Part model, mm, in its own coordinate system. A direction names the side the tool comes from. Give positions to 0.01 mm unless a question says otherwise; leave off trailing zeros. Write each loop counter-clockwise with the first axis right and the second up, starting at its lowest first coordinate (ties: lowest second). Pieces come first, ordered by that corner, then holes.
```python
from build123d import *

# Parameters (mm, degrees)
EXTRUDE_THIN1_DEPTH = 756.30962295
SKETCH2_R           = 45
EXTRUDE1_DEPTH      = 3
LPATTERN1_COUNT     = 7
LPATTERN1_PITCH     = 115
LPATTERN2_COUNT     = 7
LPATTERN2_PITCH     = 115
SKETCH3_R           = 3.175
EXTRUDE2_DEPTH      = 111


with BuildPart() as part:
    # Sketch1 → Extrude-Thin1 (new body, symmetric)
    with BuildSketch(Plane.XY):
        with BuildLine():
            Line((25.4, 55), (2.54, 55))
            ThreePointArc((2.54, 55), (0.743948776, 54.256051224), (0, 52.46))
            Line((0, 52.46), (0, -52.46))
            ThreePointArc((0, -52.46), (0.743948776, -54.256051224), (2.54, -55))
            Line((2.54, -55), (25.4, -55))
            Line((25.4, -55), (25.4, -53))
            Line((25.4, -53), (2.54, -53))
            ThreePointArc((2.54, -53), (2.158162338, -52.841837662), (2, -52.46))
            Line((2, -52.46), (2, 52.46))
            ThreePointArc((2, 52.46), (2.158162338, 52.841837662), (2.54, 53))
            Line((2.54, 53), (25.4, 53))
            Line((25.4, 53), (25.4, 55))
        make_face()
    extrude(amount=EXTRUDE_THIN1_DEPTH, both=True)

    # Sketch2 → Extrude1 (cut, through all)
    with BuildSketch(Plane(origin=(2, 0, 0), x_dir=(0, 0, -1), z_dir=(1, 0, 0))):
        Circle(SKETCH2_R)
    extrude1 = extrude(amount=-EXTRUDE1_DEPTH, mode=Mode.SUBTRACT)

    # LPattern1: Extrude1 ×7
    with Locations(*[(0, 0, i * LPATTERN1_PITCH) for i in range(1, LPATTERN1_COUNT)]):
        add(extrude1, mode=Mode.SUBTRACT)

    # LPattern2: Extrude1 ×7
    with Locations(*[(0, 0, -i * LPATTERN2_PITCH) for i in range(1, LPATTERN2_COUNT)]):
        add(extrude1, mode=Mode.SUBTRACT)

    # Sketch3 → Extrude2 (cut, through all)
    with BuildSketch(Plane.XZ.offset(55)):
        with Locations(Location((12.7, 743.60962295, 0), (0, 0, 270))):  # turned: the seam where the file's is
            Circle(SKETCH3_R)
    extrude2 = extrude(amount=-EXTRUDE2_DEPTH, mode=Mode.SUBTRACT)

    # Mirror1: Extrude2 across plane
    add(extrude2.mirror(Plane.XY), mode=Mode.SUBTRACT)


solid = part.part
```
1) Saw through at C-C, the plane z = -365. Write the cut outline in (x, y), then the cut area to 3 significant figures.
Answers follow:
outline: (0, -52.46) arc R2.54 ccw to (2.54, -55) - (25.4, -55) - (25.4, -53) - (2.54, -53) arc R0.54 cw to (2, -52.46) - (2, -40.31) - (0, -40.31) - close; (0, 40.31) - (2, 40.31) - (2, 52.46) arc R0.54 cw to (2.54, 53) - (25.4, 53) - (25.4, 55) - (2.54, 55) arc R2.54 ccw to (0, 52.46) - close
area: 150 mm2
2) Pin check, flat tip, straight feed: pin 1 Ø1.5 at (y, z) = (35, -530) entering from +X. Stop position of the tip, or through.
Answers follow:
pin 1: stops at x = 2
3) Two-plate mould, pull along Y, no slides. Class faces 1 (the face through (1, -27, 266)), 2 (the face through (1, -27, -194)), 3 (the face through (0, 47, 11)), 4 (the face through (14, -55, 11)): +Y half, -Y half, draft (parallel to the pull), parting line (faces both ways), or undercut.
Answers follow:
face 1: undercut
face 2: undercut
face 3: draft
face 4: -Y half
4) Saw through at B-B, the plane y = 22. Count the separate pieces of the cut face and the enclosed holes in it, then the cut area to 3 significant figures.
Answers follow:
separate pieces: 14
enclosed holes: 0
area: 984 mm2
5) Saw through at A-A, the plane z = 0. Write the cut outline in (x, y), then the cut area to 3 significant figures.
Answers follow:
outline: (0, -52.46) arc R2.54 ccw to (2.54, -55) - (25.4, -55) - (25.4, -53) - (2.54, -53) arc R0.54 cw to (2, -52.46) - (2, -45) - (0, -45) - close; (0, 45) - (2, 45) - (2, 52.46) arc R0.54 cw to (2.54, 53) - (25.4, 53) - (25.4, 55) - (2.54, 55) arc R2.54 ccw to (0, 52.46) - close
area: 131 mm2
6) Wall check: L1, parallel to Y at x = 2.75, z = 292.5; L2, parallel to Y at x = 1.6, z = -230; L3, parallel to X at y = 1.5, z = -285. Give the ranges that are in metal, low to high.
Answers follow:
L1: y = -55 to -53, 53 to 55
L2: y = -54.82 to -45, 45 to 54.82
L3: x = 0 to 2
7) 3-axis set-ups, long thin cutter, end or side, ignore diameter. For faces 5 (the face through (14, -53, 11)), 6 (the face through (1, -27, 151)): which of +Z, -Z, +X, -X, +Y, -Y reach the whole face in a straight line?
Answers follow:
face 5: +Z, -Z, +X
face 6: +X, -X
